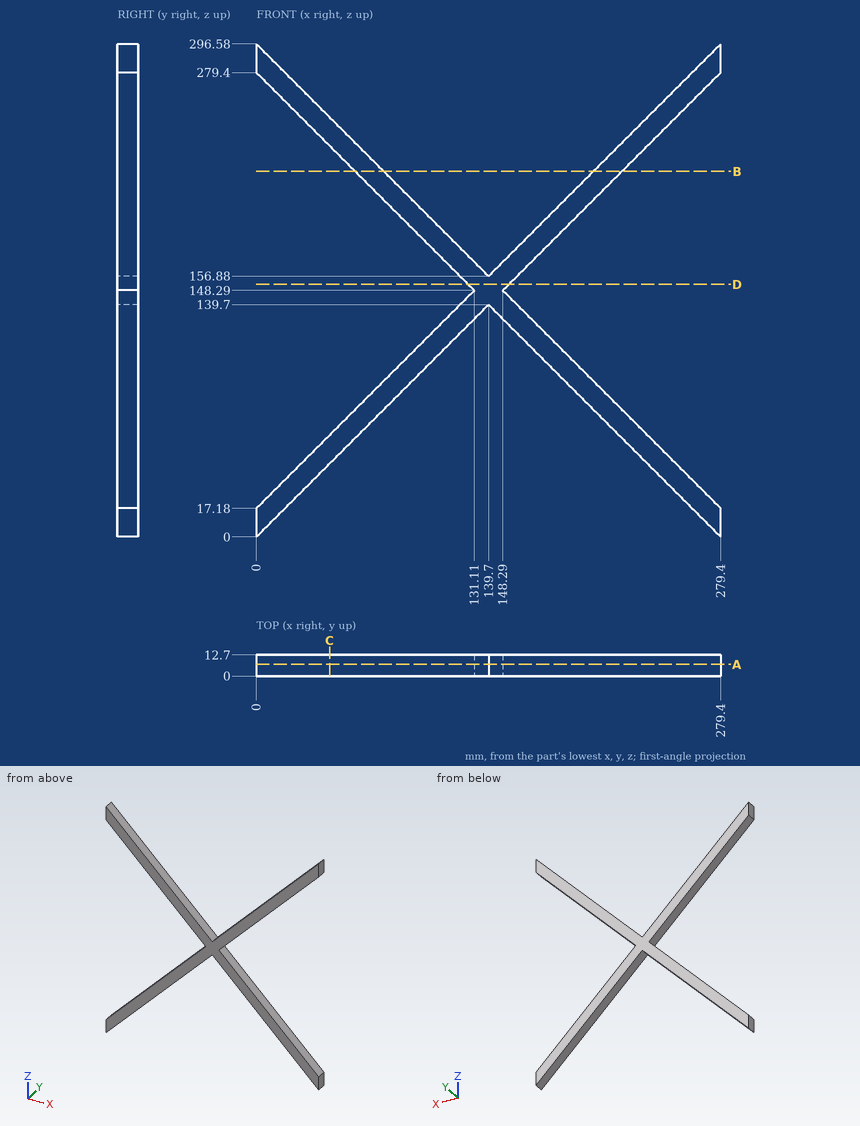
Source: three-view drawing plus pictorial views. Frame: mm from the lowest corner of the part. Coordinates: 2 decimals unless noted, no trailing zeros. Loops run counter-clockwise (first coordinate to the right, second up) from the corner with the lowest first, then second, coordinate; pieces in that order, holes last. Notation, with made-up numbers: (74.5, 53.5) -> (96.5, 53.5) arc R27 ccw to (96.5, 73.5) -> close; hole circle Ø6 at (20, 28). An arc over 180 degrees is marked (long way). One line per item, written item: value.
(1) Ray query, line 1 along X through (y, z) = (8.75, 85); line 2 along X through (y, z) = (10, 203); line 3 along Z through (x, y) = (28, 10.5). Return the intervals inside material, ascending.
Answer below:
line 1: x = 67.82 to 85, 194.4 to 211.58
line 2: x = 76.4 to 93.58, 185.82 to 203
line 3: z = 28 to 45.18, 251.4 to 268.58
(2) Cut plane C-C (x = 44). Output: boundary loops of the cut face in (y, z).
Answer below:
outline: (0, 44) -> (12.7, 44) -> (12.7, 61.18) -> (0, 61.18) -> close; (0, 235.4) -> (12.7, 235.4) -> (12.7, 252.58) -> (0, 252.58) -> close
(3) Pin query (flat end, axial travel): pin 1 Ø1.5 at (x, y) = (226, 1.5) entering from -Z; pin 2 Ø6 at (y, z) = (2.5, 114.5) entering from -X; pin 3 Ø2 at (x, y) = (190.5, 2) entering from -Z. Return the tip coordinate at first contact, or that it passes through.
Answer below:
pin 1: stops at z = 52.65
pin 2: stops at x = 94.32
pin 3: stops at z = 87.9
(4) Cut plane D-D (z = 152). Output: boundary loops of the cut face in (x, y).
Answer below:
outline: (127.4, 0) -> (152, 0) -> (152, 12.7) -> (127.4, 12.7) -> close
(5) Cut plane A-A (y = 7). Output: boundary loops of the cut face in (x, z), then the cut area to 3 significant figures.
Answer below:
outline: (0, 0) -> (139.7, 139.7) -> (279.4, 0) -> (279.4, 17.18) -> (148.29, 148.29) -> (279.4, 279.4) -> (279.4, 296.58) -> (139.7, 156.88) -> (0, 296.58) -> (0, 279.4) -> (131.11, 148.29) -> (0, 17.18) -> close
area: 9,450 mm2
(6) Cut plane B-B (z = 220). Output: boundary loops of the cut face in (x, y).
Answer below:
outline: (59.4, 0) -> (76.58, 0) -> (76.58, 12.7) -> (59.4, 12.7) -> close; (202.82, 0) -> (220, 0) -> (220, 12.7) -> (202.82, 12.7) -> close
